The model under review builds one solid part; all positions refer to its coordinate system, in mm. Face numbers are marked on the shaded views. A direction names the side the tool comes from. Coordinates: 2 decimals unless noted, no trailing zeros. Loops run counter-clockwise (first coordinate to the right, second up) from the corner with the lowest first, then second, coordinate; pieces in that order, holes last. Notation, with made-up numbers: (29, 84.25) - (54, 84.25) arc R15 cw to (54, 97.25) - close; hole circle Ø8 at (66.25, -15.5). An arc over 180 degrees is marked (long way). Use a Markdown table: item, result. Add a question column.
1) To check wall thickness, follow L1, parallel to Z at x = 10.75, y = -15; L2, parallel to Z at x = 10, y = 2; L3, parallel to Y at x = 7.75, z = 8.5. State the ranges of each line that lie inside material, in increasing order. Write a range as [from, to].
2) The part is to be moulded in two halves that separate along Y. For the marked faces 5, 6 and 7, say which applies: pulls with the +Y half, pulls with the -Y half, needs draft (parallel to the pull), parting line crosses it, or undercut.
3) Add section A-A, the plane y = -3. Give the boundary of the cut face in (x, z).
4) Add section D-D, the plane x = 4.85. Give the boundary of the cut face in (y, z), and give its area (3 significant figures).
5) Clearance check with flat-ended pins moving along their axes: pin 1 (2.5 mm diameter, centred on x = 8, y = 3, fed in from +Z); pin 2 (7 mm diameter, centred on x = 8.5, y = -17, fed in from +Z); pin 3 (3 mm diameter, centred on y = 2, z = 4, fed in from +X); pin 4 (4 mm diameter, centred on x = 13.5, z = 14.5, fed in from +Y). State where each tip first meets the part, or that it passes through.
6) Add section C-C, the plane z = 1.5. Give the boundary of the cut face in (x, y), and give its area (3 significant figures).
7) For the marked faces 1, 2, 3 and 4, list the 3-axis set-ups (+Z, -Z, +X, -X, +Y, -Y) from which the entire face can be reached by the end or side of a thin tool; tool diameter is ignored.
8) Add section B-B, the plane x = 18.25. Give the boundary of the cut face in (y, z).
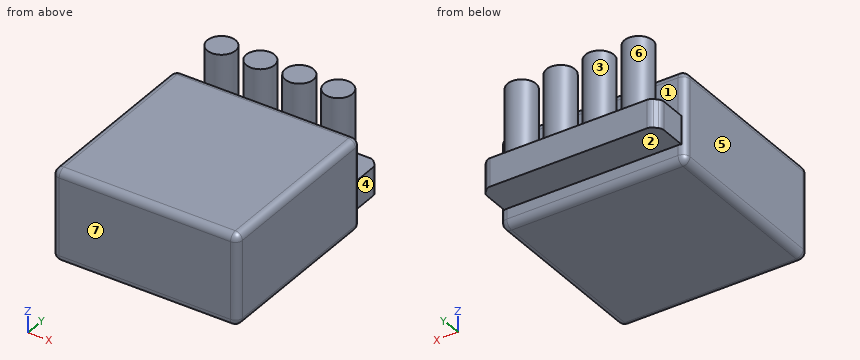
Autodesk Inventor part; units mm, degrees
ref_plane "作業平面1" through (0, 0, 6.45) normal (0, 0, 1) x (1, 0, 0)
ref_plane "YZ Plane" through (0, 0, 0) normal (1, 0, 0) x (0, 1, 0)
ref_plane "XZ Plane" through (0, 0, 0) normal (0, 1, 0) x (-1, 0, 0)
sketch "スケッチ1" plane through (0, 0, 0) normal (0, 0, 1) x (1, 0, 0)
  line L0 (0, 0) -> (26.2, 0)
  line L1 (26.2, 0) -> (26.2, -25.7)
  line L2 (26.2, -25.7) -> (0, -25.7)
  line L3 (0, -25.7) -> (0, 0)
  dimension "d0" = 25.7
  dimension "d1" = 26.2
extrude "外形" add sketch "スケッチ1" along normal blind 12.9
ref_plane "作業平面1" through (0, 0, 6.45) normal (0, 0, 1) x (1, 0, 0)
sketch "スケッチ2" plane through (0, 0, 6.45) normal (0, 0, 1) x (1, 0, 0)
  line L0 (0, 0) -> (26.2, 0)
  line L1 (0, 0) -> (26.2, 0)
  line L2 (0.6, 0) -> (0.6, 5)
  line L3 (0.6, 5) -> (25.6, 5)
  line L4 (25.6, 5) -> (25.6, 0)
  line L5 (13.1, 0) -> (13.1, 3.4882)
  dimension "d5" = 5
  dimension "d6" = 25
extrude "突起部" add sketch "スケッチ2" against normal blind 4
chamfer "面取り1" distance 1 angle 45 2 edges at (0.6, 5, 4.45) (25.6, 5, 4.45)
fillet "フィレット1" radius 1 12 edges at (0, 0, 6.45) (0, -25.7, 6.45) (26.2, -25.7, 6.45) (13.1, -25.7, 12.9) (26.2, -12.85, 12.9) (26.2, -12.85, 0) (0, -12.85, 12.9) (13.1, 0, 12.9) (13.1, 0, 0) (13.1, -25.7, 0) (26.2, 0, 6.45) (0, -12.85, 0)
fillet "フィレット2" radius 1 4 edges at (25.6, 4, 4.45) (24.6, 5, 4.45) (1.6, 5, 4.45) (0.6, 4, 4.45)
sketch "スケッチ3" plane through (0, 0, 6.45) normal (0, 0, 1) x (1, 0, 0)
  arc A0 (2.0142, 5) -> (1.3071, 4.7071) centre (2.0142, 4) ccw
  line L0 (0.6, 4) -> (1.3071, 4.7071)
  line L1 (0.6, 4) -> (0.6, -0.0835)
  arc A1 (1, 0) -> (0.6, -0.0835) centre (1, -1) ccw
  line L2 (25.2, 0) -> (1, 0)
  arc A2 (25.6, -0.0835) -> (25.2, 0) centre (25.2, -1) ccw
  line L3 (25.6, -0.0835) -> (25.6, 3.5858)
  arc A3 (25.6, 3.5858) -> (25.3071, 4.2929) centre (24.6, 3.5858) ccw
  line L4 (24.8929, 4.7071) -> (25.3071, 4.2929)
  arc A4 (24.8929, 4.7071) -> (24.1858, 5) centre (24.1858, 4) ccw
  line L5 (24.1858, 5) -> (2.0142, 5)
  line L6 (4.85, 2.5808) -> (21.35, 2.5808)
  line L7 (13.1, 5) -> (13.1, 0.3828)
  point P0 (0, 0)
  point P1 (10.35, 2.5808)
  point P2 (15.85, 2.5808)
  dimension "d14" = 5.5
  dimension "d15" = 16.5
sketch "スケッチ4" plane through (0, 0, 6.45) normal (0, 0, 1) x (1, 0, 0)
  circle A0 centre (4.85, 2.5808) radius 2
  circle A1 centre (10.35, 2.5808) radius 2
  circle A2 centre (15.85, 2.5808) radius 2
  circle A3 centre (21.35, 2.5808) radius 2
  point P0 (0, 0)
  dimension "d16" = 4
  dimension "d17" = 4
  dimension "d18" = 4
  dimension "d19" = 4
extrude "押し出し3" add sketch "スケッチ4" along normal blind 10
properties part number "市販回路_MC402CR" material "ABS Plastic"
From the geometry:
| question | item | result |
|---|---|---|
| 1 | L1 | z = [0, 12.9] |
| 1 | L2 | z = [2.45, 16.45] |
| 1 | L3 | y = [-25.7, 0] |
| 2 | face 5 | needs draft |
| 2 | face 6 | undercut |
| 2 | face 7 | pulls with the -Y half |
| 3 | outline | (0, 1) arc R1 ccw to (1, 0) - (25.2, 0) arc R1 ccw to (26.2, 1) - (26.2, 11.9) arc R1 ccw to (25.2, 12.9) - (1, 12.9) arc R1 ccw to (0, 11.9) - close |
| 4 | outline | (-25.7, 1) arc R1 ccw to (-24.7, 0) - (-1, 0) arc R1 ccw to (0, 1) - (0, 2.45) - (5, 2.45) - (5, 6.45) - (4.58, 6.45) - (4.58, 16.45) - (0.58, 16.45) - (0.58, 6.45) - (0, 6.45) - (0, 11.9) arc R1 ccw to (-1, 12.9) - (-24.7, 12.9) arc R1 ccw to (-25.7, 11.9) - close |
| 4 | area | 391 mm^2 |
| 5 | pin 1 | stops at z = 16.45 |
| 5 | pin 2 | stops at z = 12.9 |
| 5 | pin 3 | stops at x = 25.6 |
| 5 | pin 4 | stops at y = 4.55 |
| 6 | outline | (0, -24.7) arc R1 ccw to (1, -25.7) - (25.2, -25.7) arc R1 ccw to (26.2, -24.7) - (26.2, -1) arc R1 ccw to (25.2, 0) - (1, 0) arc R1 ccw to (0, -1) - close |
| 6 | area | 672 mm^2 |
| 7 | face 1 | +Z, +X, -X |
| 7 | face 2 | -Z, +X, -X, +Y |
| 7 | face 3 | +Z |
| 7 | face 4 | +Z, -Z, +X, +Y |
| 8 | outline | (-25.7, 1) arc R1 ccw to (-24.7, 0) - (-1, 0) arc R1 ccw to (0, 1) - (0, 2.45) - (5, 2.45) - (5, 6.45) - (0, 6.45) - (0, 11.9) arc R1 ccw to (-1, 12.9) - (-24.7, 12.9) arc R1 ccw to (-25.7, 11.9) - close |
